Verification items for the finished model (mm, model axes). Face numbers are marked on the shaded views. A direction names the side the tool comes from. Coordinates: 2 decimals unless noted, no trailing zeros. Write each loop counter-clockwise with the first axis right and the second up, starting at its lowest first coordinate (ties: lowest second). Pieces come first, ordered by that corner, then holes. Notation, with made-up numbers: (-24, 37.5) - (20, 37.5) arc R23 ccw to (20, 63.5) - close; hole circle Ø8 at (85, 77). An arc over 180 degrees is marked (long way). Answer as CSV lines item,"result". Start each with the question number.
```python
from build123d import *

# Parameters (mm, degrees)
BOSS_EXTRUDE1_DEPTH = 10
BOSS_EXTRUDE2_DEPTH = 15


with BuildPart() as part:
    # Sketch1 → Boss-Extrude1 (new body)
    with BuildSketch(Plane.XY):
        with BuildLine():
            Line((0, 0), (-20, 0))
            ThreePointArc((-20, 0), (-27.071067812, -2.928932188), (-30, -10))
            Line((-30, -10), (-30, -25))
            ThreePointArc((-30, -25), (-10.375361639, -18.049566033), (0, 0))
        make_face()
    extrude(amount=BOSS_EXTRUDE1_DEPTH)

    # Sketch2 → Boss-Extrude2 (add)
    with BuildSketch(Plane.XY.offset(10)):
        with BuildLine():
            Line((0, 0), (0, -15))
            ThreePointArc((0, -15), (-2.928932188, -22.071067812), (-10, -25))
            Line((-10, -25), (-30, -25))
            ThreePointArc((-30, -25), (-19.52562419, -7.069250972), (0, 0))
        make_face()
    extrude(amount=BOSS_EXTRUDE2_DEPTH)


solid = part.part
```
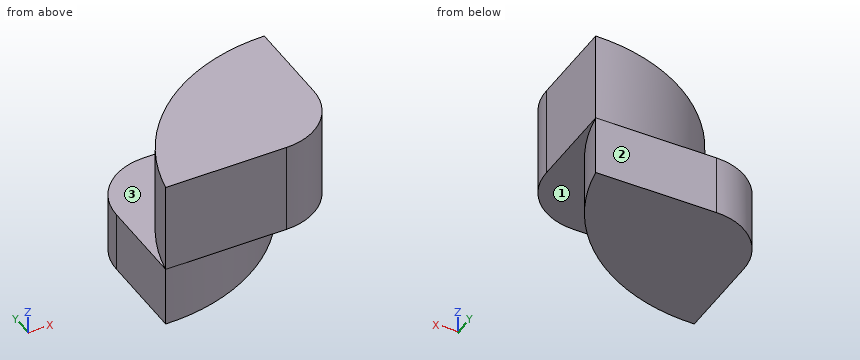
1. Depth check by flat-ended pin: P1, Ø3, axis at x = -4, z = 20.5, coming from the +Y side; P2, Ø1.5, axis at x = -10.5, z = 17, coming from the -Y side; P3, Ø8, axis at y = -14.5, z = 3.5, coming from the +X side. Enter the tip coordinate at first touch or a pass-through.
2. Cross-section at B-B (x = -25). Record the cut outline in (y, z), and give its area (3 significant figures).
3. Cross-section at C-C (z = 21). Record the cut outline in (x, y), and give its area (3 significant figures).
4. Access from +Z, -Z, +X, -X, +Y, -Y to the whole of each face (thin tool, end or side, straight path). Record for the marked faces 1, 2 and 3.
5. Cross-section at D-D (z = 2). Record the cut outline in (x, y).
6. Cross-section at A-A (y = -6). Record the cut outline in (x, z), and give its area (3 significant figures).
7. Scan lines: line 1 along Z through (x, y) = (-23, -1.5); line 2 along Z through (x, y) = (-13.5, -20.75); line 3 along Y through (x, z) = (-26, 9.25). Record each from-to range of solid material in increasing order. Write a range as from..to.
Completed:
1,P1,"stops at y = -0.1"
1,P2,"stops at y = -25"
1,P3,"stops at x = -3.89"
2,outline,"(-25, 10) - (-24.65, 10) - (-24.65, 0) - (-1.34, 0) - (-1.34, 10) - (-13.03, 10) - (-13.03, 25) - (-25, 25) - close"
2,area,"413 mm2"
3,outline,"(-30, -25) - (-10, -25) arc R10 ccw to (0, -15) - (0, 0) arc R30.5 ccw to start"
3,area,"542 mm2"
4,face 1,"-Z, +X, -Y"
4,face 2,"+Z, -Z, +X, -X, +Y"
4,face 3,"+Z, -X, +Y"
5,outline,"(-30, -25) arc R30 ccw to (0, 0) - (-20, 0) arc R10 ccw to (-30, -10) - close"
6,outline,"(-29.17, 0) - (-1.67, 0) - (-1.67, 10) - (0, 10) - (0, 25) - (-18.17, 25) - (-18.17, 10) - (-29.17, 10) - close"
6,area,"547 mm2"
7,line 1,"z = 0..10"
7,line 2,"z = 10..25"
7,line 3,"y = -24.79..-2"
